Could you check a few things on this model? Use its own coordinates, in mm. A direction names the side the tool comes from. Round coordinates to 2 decimals unless told otherwise and drop trailing zeros. Order: outer loops, then holes, each group sorted by start corner. A loop starts at its lowest first (then second) coordinate and runs counter-clockwise, first axis right, second up. Notation, with made-up numbers: (84, 62) -> (92, 62) arc R30 ccw to (92, 100) -> close; hole circle Ø11 at (81.25, -28.75). An arc over 180 degrees is marked (long way). Put each result on its own line as item: value. Start each with the question number.
Autodesk Inventor part; units mm, degrees
ref_plane "YZ Plane" through (0, 0, 0) normal (1, 0, 0) x (0, 1, 0)
ref_plane "XZ Plane" through (0, 0, 0) normal (0, 1, 0) x (-1, 0, 0)
ref_plane "XY Plane" through (0, 0, 0) normal (0, 0, 1) x (1, 0, 0)
sketch "Sketch1" plane through (0, 0, 0) normal (0, 1, 0) x (-1, 0, 0)
  circle A0 centre (0, 0) radius 6
  dimension "d0" = 12
extrude "Extrusion1" add sketch "Sketch1" along normal blind 5
sketch "Sketch2" plane through (0, 5, 0) normal (0, 1, 0) x (1, 0, 0)
  circle A0 centre (0, 0) radius 6
  circle A1 centre (0, 0) radius 6.5
  dimension "d3" = 13
extrude "Extrusion2" add sketch "Sketch2" along normal blind 0.5 contours A0 | A1
chamfer "Chamfer1" distance 0.25 angle 45 1 edges at (-6.5, 5.5, 0)
sketch "Sketch3" plane through (0, 5.5, 0) normal (0, 1, 0) x (1, 0, 0)
  circle A0 centre (0, 0) radius 6.25
  circle A1 centre (0, 0) radius 3
  dimension "d9" = 6
extrude "Extrusion3" cut sketch "Sketch3" against normal through all contours A1
properties part number "500-125" material "ABS Plastic"
1. If we section it at A-A, the plane z = 0: Please give me the cut outline in (x, y), then the cut area to 3 significant figures.
2. For pin 1 Ø2 at (x, z) = (3, 5) entering from -Y; pin 2 Ø5 at (x, z) = (0, 0) entering from +Y, each with a flat end and sliding along its axis, tell me the tip position at first contact or that it passes through.
3. Thinking about a two-plate mould opening in Z: for faces 1 (the face through (3, 0, -1)), 2 (the face through (6, 2, 0)), 3 (the face through (-3, 3, 0)), which applies, +Z half, -Z half, draft (parallel to the pull), parting line (faces both ways), or undercut?
4. I need wall thicknesses on L1, parallel to Z at x = 0, y = 1.75; L2, parallel to Z at x = 1.25, y = 3.85; L3, parallel to X at y = 3.5, z = 1.5. Which ranges of each line are inside material? Lowest first, please.
5. Which directions (+Z, -Z, +X, -X, +Y, -Y) give clear straight access to the entire face, cutting with the end or side of a thin tool? Please do faces 4 (the face through (2, 5, 6)), 5 (the face through (-1, 5.5, 3)).
6. If we section it at C-C, the plane y = 4.75: Please give me the cut outline in (x, z), then the cut area to 3 significant figures.
7. If we section it at B-B, the plane x = 0: Please give me the cut outline in (y, z).
Results below:
1. outline: (-6.5, 5) -> (-6, 5) -> (-6, 0) -> (-3, 0) -> (-3, 5.5) -> (-6.25, 5.5) -> (-6.5, 5.25) -> close; (3, 0) -> (6, 0) -> (6, 5) -> (6.5, 5) -> (6.5, 5.25) -> (6.25, 5.5) -> (3, 5.5) -> close
1. area: 33.4 mm2
2. pin 1: y = 0
2. pin 2: through
3. face 1: draft
3. face 2: parting line
3. face 3: undercut
4. L1: -6 to -3, 3 to 6
4. L2: -5.87 to -2.73, 2.73 to 5.87
4. L3: -5.81 to -2.6, 2.6 to 5.81
5. face 4: -Y
5. face 5: +Z, -Z, +X, -X, +Y
6. outline: circle Ø12 at (0, 0); hole circle Ø6 at (0, 0)
6. area: 84.8 mm2
7. outline: (0, -6) -> (5, -6) -> (5, -6.5) -> (5.25, -6.5) -> (5.5, -6.25) -> (5.5, -3) -> (0, -3) -> close; (0, 3) -> (5.5, 3) -> (5.5, 6.25) -> (5.25, 6.5) -> (5, 6.5) -> (5, 6) -> (0, 6) -> close
